from build123d import *

# Parameters (mm, degrees)
BOX012_W          = 17
BOX012_H          = 14.6
BOX012_DEPTH      = 16.5
CYLINDER025_R     = 2.1
CYLINDER025_DEPTH = 2
CYLINDER024_R     = 2.1
CYLINDER024_DEPTH = 2
CYLINDER027_R     = 3.5
CYLINDER027_DEPTH = 0.75
BOX011_W          = 7
BOX011_H          = 35
BOX011_DEPTH      = 0.75
CYLINDER026_R     = 3.5
CYLINDER026_DEPTH = 0.75
CYLINDER022_R     = 4.5
CYLINDER022_DEPTH = 1.5
CYLINDER021_R     = 14
CYLINDER021_DEPTH = 19
BOX014_W          = 1
BOX014_H          = 5
BOX014_DEPTH      = 6
BOX013_W          = 1
BOX013_H          = 5
BOX013_DEPTH      = 6
CYLINDER023_R     = 2.5
CYLINDER023_DEPTH = 8.5
CYLINDER020_R     = 5
CYLINDER020_DEPTH = 9
CYLINDER019_R     = 50
CYLINDER019_DEPTH = 2.5


with BuildPart() as cube012:
    # Box012 → Box012 (new body)
    with BuildSketch(Plane(origin=(0, -7.3, 2.5), x_dir=(1, 0, 0), z_dir=(0, 0, 1))):
        with Locations((8.5, 7.3)):
            Rectangle(BOX012_W, BOX012_H)
    extrude(amount=BOX012_DEPTH)


with BuildPart() as cylinder025:
    # Cylinder025 → Cylinder025 (new body)
    with BuildSketch(Plane(origin=(0, 17.5, 18), x_dir=(1, 0, 0), z_dir=(0, 0, 1))):
        Circle(CYLINDER025_R)
    extrude(amount=CYLINDER025_DEPTH)


with BuildPart() as cylinder024:
    # Cylinder024 → Cylinder024 (new body)
    with BuildSketch(Plane(origin=(0, -17.5, 18), x_dir=(1, 0, 0), z_dir=(0, 0, 1))):
        Circle(CYLINDER024_R)
    extrude(amount=CYLINDER024_DEPTH)


with BuildPart() as cylinder027:
    # Cylinder027 → Cylinder027 (new body)
    with BuildSketch(Plane(origin=(0, 17.5, 18), x_dir=(1, 0, 0), z_dir=(0, 0, 1))):
        Circle(CYLINDER027_R)
    extrude(amount=CYLINDER027_DEPTH)


with BuildPart() as cube011:
    # Box011 → Box011 (new body)
    with BuildSketch(Plane(origin=(-3.5, -17.5, 18), x_dir=(1, 0, 0), z_dir=(0, 0, 1))):
        with Locations((3.5, 17.5)):
            Rectangle(BOX011_W, BOX011_H)
    extrude(amount=BOX011_DEPTH)


with BuildPart() as cut010:
    # Cylinder026 → Cylinder026 (new body)
    with BuildSketch(Plane(origin=(0, -17.5, 18), x_dir=(1, 0, 0), z_dir=(0, 0, 1))):
        Circle(CYLINDER026_R)
    extrude(amount=CYLINDER026_DEPTH)

    # Fusion005: union Cylinder027, Cube011
    add(cylinder027.part)
    add(cube011.part)


with BuildPart() as cut010_1:
    # Fusion005 placement: moved
    add(cut010.part.moved(Location((0, 0, 0.25))))

    # Cut009: cut Cylinder024
    add(cylinder024.part, mode=Mode.SUBTRACT)

    # Cut010: cut Cylinder025
    add(cylinder025.part, mode=Mode.SUBTRACT)


with BuildPart() as cylinder022:
    # Cylinder022 → Cylinder022 (new body)
    with BuildSketch(Plane(origin=(-8, 0, 19), x_dir=(1, 0, 0), z_dir=(0, 0, 1))):
        Circle(CYLINDER022_R)
    extrude(amount=CYLINDER022_DEPTH)


with BuildPart() as cylinder021:
    # Cylinder021 → Cylinder021 (new body)
    with BuildSketch(Plane.XY):
        Circle(CYLINDER021_R)
    extrude(amount=CYLINDER021_DEPTH)


with BuildPart() as cube014:
    # Box014 → Box014 (new body)
    with BuildSketch(Plane(origin=(-10.5, -2.5, 23), x_dir=(1, 0, 0), z_dir=(0, 0, 1))):
        with Locations((0.5, 2.5)):
            Rectangle(BOX014_W, BOX014_H)
    extrude(amount=BOX014_DEPTH)


with BuildPart() as cube013:
    # Box013 → Box013 (new body)
    with BuildSketch(Plane(origin=(-6.5, -2.5, 23), x_dir=(1, 0, 0), z_dir=(0, 0, 1))):
        with Locations((0.5, 2.5)):
            Rectangle(BOX013_W, BOX013_H)
    extrude(amount=BOX013_DEPTH)


with BuildPart() as fusion006:
    # Cylinder023 → Cylinder023 (new body)
    with BuildSketch(Plane(origin=(-8, 0, 20.5), x_dir=(1, 0, 0), z_dir=(0, 0, 1))):
        Circle(CYLINDER023_R)
    extrude(amount=CYLINDER023_DEPTH)

    # Cut011: cut Cube013
    add(cube013.part, mode=Mode.SUBTRACT)

    # Cut012: cut Cube014
    add(cube014.part, mode=Mode.SUBTRACT)

    # Fusion006: union Cube012, Cut010, Cylinder022, Cylinder021
    add(cube012.part)
    add(cut010_1.part)
    add(cylinder022.part)
    add(cylinder021.part)


with BuildPart() as fusion006_1:
    # Fusion006 placement: moved
    add(fusion006.part.moved(Location((8, 0, -10))))


with BuildPart() as cut013:
    # Cylinder020 → Cylinder020 (new body)
    with BuildSketch(Plane.XY.offset(11)):
        Circle(CYLINDER020_R)
    extrude(amount=CYLINDER020_DEPTH)

    # Cut013: cut Fusion006
    add(fusion006_1.part, mode=Mode.SUBTRACT)


with BuildPart() as bottom_plate:
    # Cylinder019 → Cylinder019 (new body)
    with BuildSketch(Plane.XY.offset(20)):
        Circle(CYLINDER019_R)
    extrude(amount=CYLINDER019_DEPTH)

    # Fusion007: union Cut013
    add(cut013.part)


solid = bottom_plate.part
Read the model definition and answer for the solid it produces. Units are mm, in the model's axes. A direction names the side the tool comes from. Round coordinates to 2 decimals unless told otherwise and drop trailing zeros. Loops run counter-clockwise (first coordinate to the right, second up) from the corner with the lowest first, then second, coordinate; pieces in that order, holes last.
Q1. Section A-A on y = 0 is taken. Write down the section's boundary in (x, z).
Q2. Section B-B on x = 0 is taken. Write down the section's boundary in (y, z).
Q3. Which of the six approach directions +Z, -Z, +X, -X, +Y, -Y give full straight-line access (tool end or side, diameter ignored) to faces 5 (the face through (1.34, 2.11, 14.06)), 6 (the face through (2, -2, 11))?
Q4. Consider probe 1 along Y at (x, z) = (0, 14); probe 2 along Z at (x, y) = (-24, 6.5); probe 3 along X at (y, z) = (-2, 18.5). Determine where each line is inside the solid, lowest interval first.
Q5. Section D-D on y = 42 is taken. Write down the section's boundary in (x, z).
Q6. Section C-C on x = -38 is taken. Write down the section's boundary in (y, z).
Q7. Each of these flat-tipped pins is pushed along its axis until it touches: pin 1 (6 mm diameter, centred on y = 37.5, z = 21, fed in from +X); pin 2 (2 mm diameter, centred on x = 33, z = 20.5, fed in from +Y); pin 3 (5 mm diameter, centred on y = -35, z = 20.5, fed in from +X). Where does it stop, or does it pass through?
Q8. Determine the mould class of faces 1 (the face through (0, 0, 19)), 2 (the face through (-1.08, -4.88, 15.44)), 3 (the face through (1.5, 0, 16)), 4 (the face through (-1, -10, 20)) for opening direction Y: released by +Y, released by -Y, zero draft, split by the parting line, or undercut.
Output:
1. outline: (-50, 20) - (-5, 20) - (-5, 11) - (-2.5, 11) - (-2.5, 13) - (-1.5, 13) - (-1.5, 19) - (1.5, 19) - (1.5, 13) - (2.5, 13) - (2.5, 11) - (5, 11) - (5, 20) - (50, 20) - (50, 22.5) - (-50, 22.5) - close
2. outline: (-50, 20) - (-5, 20) - (-5, 11) - (-2.5, 11) - (-2.5, 19) - (2.5, 19) - (2.5, 11) - (5, 11) - (5, 20) - (50, 20) - (50, 22.5) - (-50, 22.5) - close
3. face 5: -Z
3. face 6: -Z, +X, -X, +Y, -Y
4. probe 1: y = -5 to -2.5, 2.5 to 5
4. probe 2: z = 20 to 22.5
4. probe 3: x = -4.58 to -1.5, 1.5 to 4.58
5. outline: (-27.13, 20) - (27.13, 20) - (27.13, 22.5) - (-27.13, 22.5) - close
6. outline: (-32.5, 20) - (32.5, 20) - (32.5, 22.5) - (-32.5, 22.5) - close
7. pin 1: stops at x = 36.19
7. pin 2: stops at y = 38.42
7. pin 3: stops at x = 38
8. face 1: undercut
8. face 2: split by the parting line
8. face 3: undercut
8. face 4: zero draft
